Work out the finished part from the listing and answer in its coordinate system (mm). Give positions to 0.01 mm unless a question says otherwise; leave off trailing zeros. Order: outer loops, then holes, each group sorted by start corner. A loop starts at its lowest first (then second) coordinate and runs counter-clockwise, first axis right, second up. Notation, with made-up numbers: (77, -35.5) - (110, -35.5) arc R16 ccw to (110, -12.5) - close; hole circle Ø2 at (44.25, 46.5). An arc over 180 degrees is marked (long way). Return JSON: item names as keys, results as strings. Group by question number.
from build123d import *


with BuildPart() as part:
    # Sketch1 → Revolve1 (revolve)
    with BuildSketch(Plane.XY):
        with BuildLine():
            Line((0, 7), (0, 8.848612181))
            ThreePointArc((0, 8.848612181), (-0.021453987, 8.993504255), (-0.083974853, 9.125962279))
            Line((-0.083974853, 9.125962279), (-2, 12))
            Line((-2, 12), (-2.359611797, 12))
            ThreePointArc((-2.359611797, 12), (-2.753714516, 11.807706105), (-2.844683047, 11.378732187))
            Line((-2.844683047, 11.378732187), (-2.155316953, 8.621267813))
            ThreePointArc((-2.155316953, 8.621267813), (-2.246285484, 8.192293895), (-2.640388203, 8))
            Line((-2.640388203, 8), (-3.5, 8))
            ThreePointArc((-3.5, 8), (-3.853553391, 7.853553391), (-4, 7.5))
            Line((-4, 7.5), (-4, 7))
            Line((-4, 7), (0, 7))
        make_face()
    revolve(axis=Axis((0, 0, 0), (-1, 0, 0)))


solid = part.part
1. The part is cut by section C-C (x = -1.3). Give the vertices of the cut face in (y, z), and give its area (3 significant figures).
2. Consider probe 1 along Z at (x, y) = (-2.9, 0); probe 2 along Y at (x, z) = (-1.55, 0) (3 decimals). Determine where each line is inside the solid, lowest interval first. Write a range as from..to.
3. Determine the mould class of faces 1 (the cylindrical face through (-2.18, -11.99, -0.53)), 2 (the flat face through (-4, 7, -2)), 3 (the cylindrical face through (-3.08, -1.73, 7.81)) for opening direction Y: released by +Y, released by -Y, zero draft, split by the parting line, or undercut.
4. The part is cut by section A-A (y = 0). Give the vertices of the cut face in (x, z).
5. Each of these flat-tipped pins is pushed along its axis until it touches: pin 1 (1.5 mm diameter, centred on x = -2, y = -6, fed in from -Z); pin 2 (1 mm diameter, centred on x = -1, y = -5, fed in from +Z). Where does it stop, or does it pass through?
Answers:
{
 "1": {"outline": "circle Ø21.9 at (0, 0); hole circle Ø14 at (0, 0)", "area": "223 mm^2"},
 "2": {"probe 1": "z = -8..-7, 7..8", "probe 2": "y = -11.325..-7, 7..11.325"},
 "3": {"face 1": "split by the parting line", "face 2": "zero draft", "face 3": "undercut"},
 "4": {"outline": "(-4, -7.5) arc R0.5 ccw to (-3.5, -8) - (-2.64, -8) arc R0.5 cw to (-2.16, -8.62) - (-2.84, -11.38) arc R0.5 ccw to (-2.36, -12) - (-2, -12) - (-0.08, -9.13) arc R0.5 ccw to (0, -8.85) - (0, -7) - (-4, -7) - close; (-4, 7) - (0, 7) - (0, 8.85) arc R0.5 ccw to (-0.08, 9.13) - (-2, 12) - (-2.36, 12) arc R0.5 ccw to (-2.84, 11.38) - (-2.16, 8.62) arc R0.5 cw to (-2.64, 8) - (-3.5, 8) arc R0.5 ccw to (-4, 7.5) - close"},
 "5": {"pin 1": "stops at z = -10.79", "pin 2": "stops at z = 10.11"}
}
